Read the model definition and answer for the solid it produces. Units are mm, in the model's axes. Face numbers are marked on the shaded views. A direction names the side the tool comes from. Give positions to 0.01 mm unless a question says otherwise; leave off trailing zeros. Order: outer loops, then holes, each group sorted by start corner. A loop starts at its lowest first (then second) coordinate and runs counter-clockwise, first axis right, second up. Notation, with made-up numbers: (50, -4.5) - (94, -4.5) arc R18 cw to (94, 9.5) - close; hole circle Ø4 at (8, 62.25). An arc over 180 degrees is marked (long way). Write item = value, one per line.
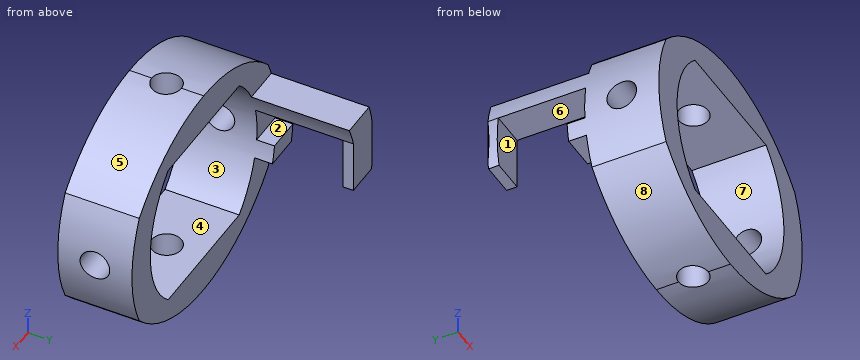
Autodesk Inventor part; units mm, degrees
ref_plane "YZ Plane" through (0, 0, 0) normal (1, 0, 0) x (0, 1, 0)
ref_plane "XZ Plane" through (0, 0, 0) normal (0, 1, 0) x (-1, 0, 0)
ref_plane "XY Plane" through (0, 0, 0) normal (0, 0, 1) x (1, 0, 0)
sketch "Sketch1" plane through (0, 0, 0) normal (0, 1, 0) x (-1, 0, 0)
  line L0 (-22.2991, -25) -> (22.2991, -25)
  line L1 (22.2991, 25) -> (-22.2991, 25)
  arc A0 (-22.2991, 25) -> (-22.2991, -25) centre (0, 0) ccw
  arc A1 (22.2991, -25) -> (22.2991, 25) centre (0, 0) ccw
  line L2 (24.8747, 37.5) -> (-24.8747, 37.5)
  line L3 (24.8747, -37.5) -> (-24.8747, -37.5)
  arc A2 (24.8747, -37.5) -> (24.8747, 37.5) centre (0, 0) ccw
  arc A3 (-24.8747, 37.5) -> (-24.8747, -37.5) centre (0, 0) ccw
  circle A4 centre (0, 0) radius 25 construction
  arc A5 (0, 37.5) -> (-40.3994, 19.8214) centre (0, -17.5) ccw
  arc A6 (40.3994, 19.8214) -> (0, 37.5) centre (0, -17.5) ccw
  arc A7 (-40.3994, -19.8214) -> (0, -37.5) centre (0, 17.5) ccw
  arc A8 (0, -37.5) -> (40.3994, -19.8214) centre (0, 17.5) ccw
  point P0 (-40.0764, 20.168)
  point P1 (-40.0764, -20.168)
  point P2 (40.0764, 20.168)
  point P3 (40.0764, -20.168)
  dimension "d2" = 50
  dimension "d3" = 33.5
  dimension "d4" = 33.5
  dimension "d5" = 44.5982
  dimension "d7" = 12.5
  dimension "d8" = 12.5
  dimension "d54" = 45
  dimension "d55" = 45
  dimension "d60" = 55
  dimension "d61" = 55
  dimension "d62" = 55
  dimension "d63" = 55
extrude "Extrusion1" add sketch "Sketch1" along normal mid plane 25
sketch "Sketch3" plane through (0, 0, 0) normal (0, 0, 1) x (1, 0, 0)
  circle A0 centre (0, 0) radius 5
  dimension "d13" = 10
extrude "Extrusion2" cut sketch "Sketch3" along normal through all both and the other way through all
sketch "Sketch5" plane through (0, 0, 0) normal (1, 0, 0) x (0, 1, 0)
  circle A0 centre (0, 0) radius 5
  dimension "d17" = 10
extrude "Extrusion3" cut sketch "Sketch5" along normal through all both and the other way through all
sketch "Sketch6" plane through (0, 12.5, 0) normal (0, 1, 0) x (1, 0, 0)
  circle A0 centre (0, 0) radius 25 construction
  arc A1 (-22.2991, 25) -> (-22.2991, -25) centre (0, 0) ccw
  line L0 (-33.5, 0) -> (-47.5, 0) construction
  line L1 (-42.4264, -15) -> (-29.9541, -15)
  line L2 (-31.9726, 10) -> (-43.8748, 10)
  arc A2 (-24.8747, 37.5) -> (-24.8747, -37.5) centre (0, 0) ccw
  arc A3 (-43.8748, 10) -> (-43.9189, 9.8046) centre (0, 0) ccw
  line L3 (-32.5308, -8) -> (-44.2832, -8)
  arc A4 (-33.5, 0) -> (-29.9541, -15) centre (0, 0) ccw
  arc A5 (-43.9204, -9.798) -> (-42.4264, -15) centre (0, 0) ccw
  arc A6 (-43.8748, 10) -> (-43.9204, -9.798) centre (0, 0) ccw
  arc A7 (-31.9726, 10) -> (-33.5, 0) centre (0, 0) ccw
  line L4 (-44.7214, 5) -> (-33.1248, 5)
  arc A8 (-22.2991, 25) -> (-22.2991, -25) centre (0, 0) ccw
  line L5 (-33.2603, 4) -> (-44.8219, 4)
  point P0 (-44.2832, -8)
  point P1 (-44.8219, 4)
  dimension "d25" = 50
  dimension "d26" = 25
  dimension "d27" = 7
  dimension "d28" = 15
  dimension "d29" = 15
  dimension "d30" = 24.8046
  dimension "d31" = 5.202
  dimension "d32" = 47.5
  dimension "d37" = 6
extrude "Extrusion4" add sketch "Sketch6" along normal blind 6 contours A1 L4 A2 L2 | A1 L5 A2 L4 | A1 L3 A2 L5
extrude "Extrusion5" add sketch "Sketch6" along normal blind 33 contours A1 L1 A2 L3
extrude "Extrusion6" cut sketch "Sketch6" along normal through all contours A1 L3 A2 L5
sketch "Sketch7" plane through (-32.5308, 45.5, 8) normal (0, 0, -1) x (-1, 0, 0)
  line L0 (0, 0) -> (11.7524, 0)
  line L1 (-2.5766, -33) -> (-2.5766, 0)
  line L2 (11.7524, 0) -> (0, 0)
  line L3 (0, -3.5185) -> (15.3049, -3.5185)
  line L4 (15.3049, -3.5185) -> (11.7524, 0)
  line L5 (0, 0) -> (0, -3.5185)
  line L6 (0, -33) -> (0, 0)
  point P0 (-32.5308, -45.5)
  dimension "d40" = 5
  dimension "d41" = 15.3049
extrude "Extrusion7" add sketch "Sketch7" along normal up to surface (18 mm away)
sketch "Sketch8" plane through (0, 45.5, 0) normal (0, 1, 0) x (1, 0, 0)
  circle A0 centre (0, 0) radius 45
  circle A1 centre (0, 0) radius 62.5
  dimension "d56" = 90
  dimension "d57" = 125
extrude "Extrusion8" cut sketch "Sketch8" against normal through all
extrude "Extrusion9" cut sketch "Sketch1" along normal through all both and the other way through all contours A2 A6 L2 | A5 A3 L2 | A2 L3 A8 | A7 L3 A3
1. For the marked faces 1, 2, 3 and 4, determine the directions among +Z, -Z, +X, -X, +Y, -Y from which every point of the face is accessible in a straight line to the end or side of a thin tool.
Recorded:
face_1 = -Z, +X, -X
face_2 = +X, -X
face_3 = -Y
face_4 = +Y, -Y
2. Section A-A (z = 18) is taken. Determine the outline of the cut face in (x, y), and give its area (3 significant figures).
Recorded:
outline = (-41.24, -12.5) - (-28.25, -12.5) - (-28.25, 12.5) - (-41.24, 12.5) - close; (28.25, -12.5) - (41.24, -12.5) - (41.24, 12.5) - (28.25, 12.5) - close
area = 649 mm^2
3. Section D-D (y = 0) is taken. Determine the outline of the cut face in (x, z), and give its area (3 significant figures).
Recorded:
outline = (-44.72, -5) arc R45 ccw to (-40.4, -19.82) arc R55 ccw to (-5, -37.27) - (-5, -25) - (-22.3, -25) arc R33.5 cw to (-33.12, -5) - close; (-44.72, 5) - (-33.12, 5) arc R33.5 cw to (-22.3, 25) - (-5, 25) - (-5, 37.27) arc R55 ccw to (-40.4, 19.82) arc R45 ccw to start; (5, -37.27) arc R55 ccw to (40.4, -19.82) arc R45 ccw to (44.72, -5) - (33.12, -5) arc R33.5 cw to (22.3, -25) - (5, -25) - close; (5, 25) - (22.3, 25) arc R33.5 cw to (33.12, 5) - (44.72, 5) arc R45 ccw to (40.4, 19.82) arc R55 ccw to (5, 37.27) - close
area = 1,940 mm^2
4. Straight lines are drawn through the part: L1, parallel to Y at x = -35.5, z = 0; L2, parallel to Y at x = 0, z = -30.5; L3, parallel to Z at x = 36.5, y = 0. For each, find the intervals that lie inside material, in ascending order. Write a range as [from, to].
Recorded:
L1 = [-12.5, -5], [5, 12.5], [41.98, 45.5]
L2 = [-12.5, -5], [5, 12.5]
L3 = [-23.64, -5], [5, 23.64]
5. Determine the mould class of the marked faces 5, 6, 7 and 8 for opening direction X: +X half, -X half, draft (parallel to the pull), parting line (faces both ways), or undercut.
Recorded:
face_5 = +X half
face_6 = draft
face_7 = undercut
face_8 = -X half
6. Section C-C (x = -19) is taken. Determine the outline of the cut face in (y, z), and give its area (3 significant figures).
Recorded:
outline = (-12.5, -34.11) - (12.5, -34.11) - (12.5, -25) - (-12.5, -25) - close; (-12.5, 25) - (12.5, 25) - (12.5, 34.11) - (-12.5, 34.11) - close
area = 456 mm^2
7. Section B-B (z = 0) is taken. Determine the outline of the cut face in (x, y).
Recorded:
outline = (-45, -12.5) - (-33.5, -12.5) - (-33.5, -5) - (-45, -5) - close; (-45, 5) - (-33.5, 5) - (-33.5, 12.5) - (-45, 12.5) - close; (-45, 41.98) - (-32.53, 41.98) - (-32.53, 45.5) - (-44.28, 45.5) - (-45, 44.79) - close; (33.5, -12.5) - (45, -12.5) - (45, -5) - (33.5, -5) - close; (33.5, 5) - (45, 5) - (45, 12.5) - (33.5, 12.5) - close
8. Flat-ended cylindrical pins translate along their axes: pin 1 (6 mm diameter, centred on x = -37, y = 31, fed in from -Z); pin 2 (1.8 mm diameter, centred on x = -38.5, y = 43.5, fed in from -Z); pin 3 (2 mm diameter, centred on y = 8, z = -14.5, fed in from -X). Find the tip coordinate at first contact, or state that the pin passes through.
Recorded:
pin_1 = 8
pin_2 = -10
pin_3 = -42.93
